Can you work these out from the model? Positions are in its coordinate system, mm. Face numbers are marked on the shaded views. A direction names the side the tool comes from. Coordinates: 2 decimals unless noted, no trailing zeros. Order: outer loops, then holes, each group sorted by start corner. A loop starts at its lowest first (then second) coordinate and runs counter-clockwise, first axis right, second up. Notation, with made-up numbers: (44.5, 67.5) -> (72.5, 67.5) arc R17 ccw to (72.5, 85.5) -> close; hole circle Ø7 at (-15.75, -11). An arc over 180 degrees is marked (long way). Use a Markdown table: item, result. Add a question column.
1. We'd pull the mould along Y, two halves only. Please class the marked faces 1, 2 and 3: pulls with the +Y half, pulls with the -Y half, needs draft (parallel to the pull), parting line crosses it, or undercut.
2. Suppose I cut it at C-C, the plane x = -293.5. List the corners of the cut face in (y, z) for me (3 decimals).
3. For pin 1 Ø1 at (x, z) = (-69.5, 45.5) entering from +Y; pin 2 Ø23 at (x, y) = (-15, -254.5) entering from +Z; pin 3 Ø10 at (y, z) = (142, 40.5) entering from +X, each with a flat end and sliding along its axis, tell me the tip position at first contact or that it passes through.
4. Suppose I cut it at B-B, the plane y = 0. List the corners of the cut face in (x, z) for me, then the cut area to 3 significant figures.
5. If I drill on line 1 along Y through (x, z) = (0, 88); line 2 along Y through (x, z) = (0, 122); line 3 along X through (y, z) = (-3, 18), over which ranges is the centre line in solid material (lowest first)? Write a range as from..to.
6. Suppose I cut it at D-D, the plane y = 254. List the corners of the cut face in (x, z) for me, then the cut area to 3 significant figures.
7. For the marked faces 4 and 5, which set-ups out of +Z, -Z, +X, -X, +Y, -Y let a thin tool reach every point of the face, with its end or its side?
8. Suppose I cut it at A-A, the plane x = 47.5. List the corners of the cut face in (y, z) for me.
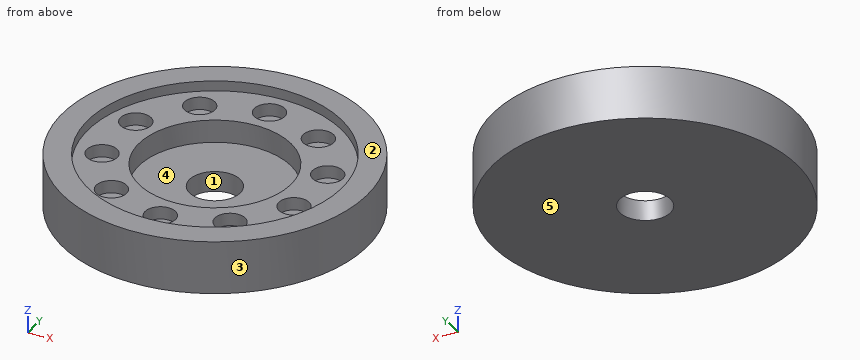
```python
from build123d import *

# Parameters (mm, degrees)
SKETCH1_R           = 381
BOSS_EXTRUDE1_DEPTH = 133.35
SKETCH2_R           = 63.5
CUT_EXTRUDE1_DEPTH  = 556.071367033
SKETCH6_R           = 317.5
CUT_EXTRUDE5_DEPTH  = 25.4
SKETCH7_R           = 190.5
CUT_EXTRUDE6_DEPTH  = 82.55
SKETCH8_R           = 38.1
CUT_EXTRUDE8_DEPTH  = 57.15


with BuildPart() as part:
    # Sketch1 → Boss-Extrude1 (new body)
    with BuildSketch(Plane.XY):
        Circle(SKETCH1_R)
    extrude(amount=BOSS_EXTRUDE1_DEPTH)

    # Sketch2 → Cut-Extrude1 (cut, through all)
    with BuildSketch(Plane.XY.offset(133.35)):
        Circle(SKETCH2_R)
    extrude(amount=-CUT_EXTRUDE1_DEPTH, mode=Mode.SUBTRACT)

    # Sketch6 → Cut-Extrude5 (cut)
    with BuildSketch(Plane.XY.offset(133.35)):
        Circle(SKETCH6_R)
    extrude(amount=-CUT_EXTRUDE5_DEPTH, mode=Mode.SUBTRACT)

    # Sketch7 → Cut-Extrude6 (cut)
    with BuildSketch(Plane.XY.offset(133.35)):
        Circle(SKETCH7_R)
    extrude(amount=-CUT_EXTRUDE6_DEPTH, mode=Mode.SUBTRACT)

    # Sketch8 → Cut-Extrude8 (cut)
    with BuildSketch(Plane.XY.offset(133.35)):
        with Locations((0, 254)):
            Circle(SKETCH8_R)
        with Locations((149.297454082, 205.490316571)):
            Circle(SKETCH8_R)
        with Locations((241.568355139, 78.490316571)):
            Circle(SKETCH8_R)
        with Locations((241.568355139, -78.490316571)):
            Circle(SKETCH8_R)
        with Locations((149.297454082, -205.490316571)):
            Circle(SKETCH8_R)
        with Locations((0, -254)):
            Circle(SKETCH8_R)
        with Locations((-149.297454082, -205.490316571)):
            Circle(SKETCH8_R)
        with Locations((-241.568355139, -78.490316571)):
            Circle(SKETCH8_R)
        with Locations((-241.568355139, 78.490316571)):
            Circle(SKETCH8_R)
        with Locations((-149.297454082, 205.490316571)):
            Circle(SKETCH8_R)
    extrude(amount=-CUT_EXTRUDE8_DEPTH, mode=Mode.SUBTRACT)


solid = part.part
```
Worked out:
| question | item | result |
|---|---|---|
| 1 | face 1 | undercut |
| 1 | face 2 | needs draft |
| 1 | face 3 | parting line crosses it |
| 2 | outline | (-242.938, 0) -> (242.938, 0) -> (242.938, 133.35) -> (121.095, 133.35) -> (121.095, 107.95) -> (-121.095, 107.95) -> (-121.095, 133.35) -> (-242.938, 133.35) -> close |
| 3 | pin 1 | stops at y = 374.7 |
| 3 | pin 2 | stops at z = 76.2 |
| 3 | pin 3 | stops at x = 355.52 |
| 4 | outline | (-381, 0) -> (-63.5, 0) -> (-63.5, 50.8) -> (-190.5, 50.8) -> (-190.5, 107.95) -> (-317.5, 107.95) -> (-317.5, 133.35) -> (-381, 133.35) -> close; (63.5, 0) -> (381, 0) -> (381, 133.35) -> (317.5, 133.35) -> (317.5, 107.95) -> (190.5, 107.95) -> (190.5, 50.8) -> (63.5, 50.8) -> close |
| 4 | area | 57,300 mm² |
| 5 | line 1 | y = -381..-292.1, -215.9..-190.5, 190.5..215.9, 292.1..381 |
| 5 | line 2 | y = -381..-317.5, 317.5..381 |
| 5 | line 3 | x = -380.99..-63.43, 63.43..380.99 |
| 6 | outline | (-283.98, 0) -> (283.98, 0) -> (283.98, 133.35) -> (190.5, 133.35) -> (190.5, 107.95) -> (38.1, 107.95) -> (38.1, 76.2) -> (-38.1, 76.2) -> (-38.1, 107.95) -> (-190.5, 107.95) -> (-190.5, 133.35) -> (-283.98, 133.35) -> close |
| 6 | area | 63,600 mm² |
| 7 | face 4 | +Z |
| 7 | face 5 | -Z, +X, -X, +Y, -Y |
| 8 | outline | (-378.03, 0) -> (-42.14, 0) -> (-42.14, 50.8) -> (-184.48, 50.8) -> (-184.48, 107.95) -> (-313.93, 107.95) -> (-313.93, 133.35) -> (-378.03, 133.35) -> close; (42.14, 0) -> (378.03, 0) -> (378.03, 133.35) -> (313.93, 133.35) -> (313.93, 107.95) -> (184.48, 107.95) -> (184.48, 50.8) -> (42.14, 50.8) -> close |
